Geometry: final body of the model. Coordinates: model frame, mm. A direction names the side the tool comes from. Coordinates: 2 decimals unless noted, no trailing zeros. Write each loop counter-clockwise with the first axis right and the second up, starting at its lowest first coordinate (ties: lowest second). Pieces come first, ordered by that corner, then holes. Notation, with made-up numbers: (51, 79.5) -> (82, 79.5) arc R21 ccw to (82, 99.5) -> close; hole circle Ø8 at (-8, -20.75). An arc over 180 degrees is marked (long way). One line per item, written item: value.
```python
from build123d import *

# Parameters (mm, degrees)
F2_W     = 28
F2_H     = 2
F2_W_2   = 2
F2_W_3   = 19.5
F2_H_2   = 19.5
F3_DEPTH = 2
F4_DEPTH = 30
F5_R     = 2
F6_DEPTH = 25
F7_R     = 2
F8_DEPTH = 25


with BuildPart() as f3:
    # F2 (on Front) → F3 (new body)
    with BuildSketch(Plane.XZ):
        with Locations((14, 1)):
            Rectangle(F2_W, F2_H)
        Polygon((28, 0), (0, 0), (0, -6.5), (6.5, -6.5), (8.5, -6.5), (28, -6.5), align=None)
        with Locations((-1, 1)):
            Rectangle(F2_W_2, F2_H)
        Polygon((0, -6.5), (0, 0), (-2, 0), (-2, -28), (0, -28), align=None)
        Polygon((6.5, -6.5), (0, -6.5), (0, -28), (6.5, -28), (6.5, -8.5), align=None)
        with Locations((18.25, -7.5)):
            Rectangle(F2_W_3, F2_H)
        with Locations((7.5, -7.5)):
            Rectangle(F2_W_2, F2_H)
        with Locations((7.5, -18.25)):
            Rectangle(F2_W_2, F2_H_2)
    extrude(amount=F3_DEPTH)

    # F2 (on Front) → F4 (join)
    with BuildSketch(Plane.XZ):
        with Locations((14, 1)):
            Rectangle(F2_W, F2_H)
        with Locations((-1, 1)):
            Rectangle(F2_W_2, F2_H)
        Polygon((0, -6.5), (0, 0), (-2, 0), (-2, -28), (0, -28), align=None)
        with Locations((18.25, -7.5)):
            Rectangle(F2_W_3, F2_H)
        with Locations((7.5, -7.5)):
            Rectangle(F2_W_2, F2_H)
        with Locations((7.5, -18.25)):
            Rectangle(F2_W_2, F2_H_2)
    extrude(amount=F4_DEPTH)

    # F5 (on face) → F6 (cut)
    with BuildSketch(Plane(origin=(0, 0, -8.5), x_dir=(1, 0, 0), z_dir=(0, 0, -1))):
        with Locations((18.25, 22.5)):
            Circle(F5_R)
        with Locations((18.25, 7.5)):
            Circle(F5_R)
    extrude(amount=-F6_DEPTH, mode=Mode.SUBTRACT)

    # F7 (on face) → F8 (cut)
    with BuildSketch(Plane.YZ.offset(8.5)):
        with Locations((-22.5, -18.25)):
            Circle(F7_R)
        with Locations((-7.5, -18.25)):
            Circle(F7_R)
    extrude(amount=-F8_DEPTH, mode=Mode.SUBTRACT)


solid = f3.part
```
(1) Section C-C (y = -7.5). Return the cut outline in (x, z).
Responses:
outline: (-2, -28) -> (0, -28) -> (0, -20.25) -> (-2, -20.25) -> close; (-2, -16.25) -> (0, -16.25) -> (0, 0) -> (16.25, 0) -> (16.25, 2) -> (-2, 2) -> close; (6.5, -28) -> (8.5, -28) -> (8.5, -20.25) -> (6.5, -20.25) -> close; (6.5, -16.25) -> (8.5, -16.25) -> (8.5, -8.5) -> (16.25, -8.5) -> (16.25, -6.5) -> (6.5, -6.5) -> close; (20.25, -8.5) -> (28, -8.5) -> (28, -6.5) -> (20.25, -6.5) -> close; (20.25, 0) -> (28, 0) -> (28, 2) -> (20.25, 2) -> close
(2) Section B-B (x = 18.25). Return the cut outline in (y, z).
Responses:
outline: (-30, -8.5) -> (-24.5, -8.5) -> (-24.5, -6.5) -> (-30, -6.5) -> close; (-30, 0) -> (-24.5, 0) -> (-24.5, 2) -> (-30, 2) -> close; (-20.5, -8.5) -> (-9.5, -8.5) -> (-9.5, -6.5) -> (-20.5, -6.5) -> close; (-20.5, 0) -> (-9.5, 0) -> (-9.5, 2) -> (-20.5, 2) -> close; (-5.5, -8.5) -> (0, -8.5) -> (0, 2) -> (-5.5, 2) -> (-5.5, 0) -> (-2, 0) -> (-2, -6.5) -> (-5.5, -6.5) -> close
(3) Reachability of faces 1 (the cylindrical face through (-0.986, -7.76, -16.267)), 2 (the flat face through (6.5, -16, -17)), 3 (the flat face through (8, -30, -12)), 4 (the flat face through (14, -16, 0)), 5 (the flat face through (8.5, -15, -18)) from +Z, -Z, +X, -X, +Y, -Y: full face, straight path, thin tool, end or side. Return the list, or none.
Responses:
face 1: +X, -X
face 2: -Z, -Y
face 3: +Z, -Z, +X, -X, -Y
face 4: +X, -Y
face 5: -Z, +X, +Y, -Y
(4) Line query: line 1 (Z direction, x = 25.5, y = -20.25); line 2 (Z direction, x = -1.1, y = -7.5); line 3 (X direction, y = -24, z = -9.5). Output: solid intervals per line, ascending. Write a range as [from, to].
Responses:
line 1: z = [-8.5, -6.5], [0, 2]
line 2: z = [-28, -20.25], [-16.25, 2]
line 3: x = [-2, 0], [6.5, 8.5]
(5) Section A-A (y = -25.25). Return the cut outline in (x, z).
Responses:
outline: (-2, -28) -> (0, -28) -> (0, 0) -> (28, 0) -> (28, 2) -> (-2, 2) -> close; (6.5, -28) -> (8.5, -28) -> (8.5, -8.5) -> (28, -8.5) -> (28, -6.5) -> (6.5, -6.5) -> close
(6) First-contact query: pin 1 (6 mm diameter, centred on y = -15.5, z = -23, fed in from +X); pin 2 (8 mm diameter, centred on x = 10.5, z = -24.5, fed in from -Y); pin 3 (6 mm diameter, centred on x = 15, y = -13.5, fed in from -Z); pin 4 (2.5 mm diameter, centred on x = 18.25, y = -7.5, fed in from -Z). Flat tips, straight axial feed; report the tip coordinate or a pass-through.
Responses:
pin 1: stops at x = 8.5
pin 2: stops at y = -30
pin 3: stops at z = -8.5
pin 4: passes through
(7) Pull-direction query (Y, two-part tool) for faces 6 (the flat face through (-0.4, -30, -6.3)), 7 (the cylindrical face through (16.776, -8.852, 0.986)), 8 (the flat face through (28, -15, -7)); classes: released by +Y, released by -Y, zero draft, split by the parting line, or undercut.
Responses:
face 6: released by -Y
face 7: undercut
face 8: zero draft
(8) Section D-D (z = -18.25). Return the cut outline in (x, y), then the cut area to 3 significant figures.
Responses:
outline: (-2, -30) -> (0, -30) -> (0, -24.5) -> (-2, -24.5) -> close; (-2, -20.5) -> (0, -20.5) -> (0, -9.5) -> (-2, -9.5) -> close; (-2, -5.5) -> (0, -5.5) -> (0, -2) -> (6.5, -2) -> (6.5, -5.5) -> (8.5, -5.5) -> (8.5, 0) -> (-2, 0) -> close; (6.5, -30) -> (8.5, -30) -> (8.5, -24.5) -> (6.5, -24.5) -> close; (6.5, -20.5) -> (8.5, -20.5) -> (8.5, -9.5) -> (6.5, -9.5) -> close
area: 101 mm2
